```python
from build123d import *

# Parameters (mm, degrees)
F3_R           = 12.5
F3_R_2         = 9.5
F3_R_3         = 7.5
F4_DEPTH       = 5
F5_DEPTH       = 40
F6_START       = 8
F6_DEPTH       = 3
F7_START       = 14
F7_DEPTH       = 3
F8_R           = 1.49999
F9_R           = 1.49999
F10_R          = 4.99999
F14_R          = 2.5
F15_DEPTH      = 2.5
F15_DEPTH_BACK = 2.5
F16_SIZE       = 4.99999


# Not quite as in the source:
# - a fillet or chamfer is up to 0.001 mm smaller than in the source, because OpenCascade refuses the exact size


with BuildPart() as f4:
    # F3 (on Top) → F4 (new body)
    with BuildSketch(Plane.XY):
        Circle(F3_R)
        Circle(F3_R_2, mode=Mode.SUBTRACT)
        Circle(F3_R_2)
        Circle(F3_R_3, mode=Mode.SUBTRACT)
        Circle(F3_R_3)
    extrude(amount=F4_DEPTH)

    # F3 (on Top) → F5 (join)
    with BuildSketch(Plane.XY):
        Circle(F3_R_3)
    extrude(amount=F5_DEPTH)

    # F3 (on Top) → F6 (join)
    with BuildSketch(Plane.XY.offset(F6_START)):
        Circle(F3_R_2)
        Circle(F3_R_3, mode=Mode.SUBTRACT)
    extrude(amount=F6_DEPTH)

    # F3 (on Top) → F7 (join)
    with BuildSketch(Plane.XY.offset(F7_START)):
        Circle(F3_R_2)
        Circle(F3_R_3, mode=Mode.SUBTRACT)
    extrude(amount=F7_DEPTH)

    # F8 (radius 1.5 in the source; OpenCascade refuses exactly that, so slightly less here)
    f8_edges = [f4.edges().sort_by_distance(p)[0] for p in [
        (-9.5, 0, 8),
        (-9.5, 0, 11),
    ]]
    fillet(f8_edges, radius=F8_R)

    # F9 (radius 1.5 in the source; OpenCascade refuses exactly that, so slightly less here)
    f9_edges = [f4.edges().sort_by_distance(p)[0] for p in [
        (-9.5, 0, 14),
        (-9.5, 0, 17),
    ]]
    fillet(f9_edges, radius=F9_R)

    # F10 (radius 5 in the source; OpenCascade refuses exactly that, so slightly less here)
    f10_edges = [f4.edges().sort_by_distance(p)[0] for p in [
        (-12.5, 0, 5),
    ]]
    fillet(f10_edges, radius=F10_R)

    # F14 (on Front) → F15 (join, two sides)
    with BuildSketch(Plane.XZ) as f15_sk:
        Polygon((-2.5, 50), (-2.5, 40), (2.5, 40), (2.5, 50), (7.5, 50), (7.5, 55), (2.5, 55), (2.5, 60), (-2.5, 60), (-2.5, 55), (-7.5, 55), (-7.5, 50), align=None)
        with Locations((0, 50.75)):
            Circle(F14_R, mode=Mode.SUBTRACT)
    extrude(amount=F15_DEPTH)
    extrude(f15_sk.sketch, amount=-F15_DEPTH_BACK)

    # F16 (size 5 in the source; OpenCascade refuses exactly that, so slightly less here)
    f16_edges = [f4.edges().sort_by_distance(p)[0] for p in [
        (-2.5, 0, 50),
        (2.5, 0, 50),
    ]]
    chamfer(f16_edges, length=F16_SIZE)


solid = f4.part
```
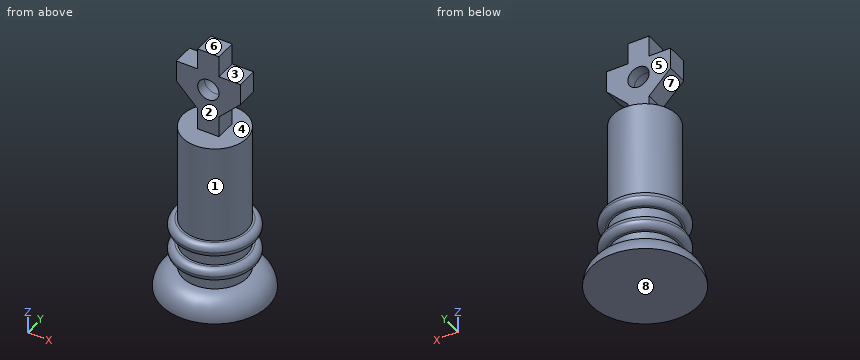
Design review of the part built by this model. Coordinates are the model's own, in mm. Face numbers are marked on the shaded views. A direction names the side the tool comes from. Coordinates: 2 decimals unless noted, no trailing zeros. Order: outer loops, then holes, each group sorted by start corner. A loop starts at its lowest first (then second) coordinate and runs counter-clockwise, first axis right, second up.
1) Wall thickness on line 1 along Z through (x, y) = (0, -1.85); line 2 along Z through (x, y) = (-1.5, -7.75); line 3 along X through (y, z) = (2.25, 45): over which ranges is each line inside the solid? List them lowest first.
2) Mouldability with a two-part tool opening along Z and no side actions: class the marked faces 1, 2 and 3 as +Z half, -Z half, draft (parallel to the pull), parting line (faces both ways), or undercut.
3) Take a section at B-B, the plane z = 43. Give the boundary of the cut face in (x, y), and give its area (3 significant figures).
4) Clearance check with flat-ended pins moving along their axes: pin 1 (5.5 mm diameter, centred on y = -0.5, z = 43.5, fed in from -X); pin 2 (7.5 mm diameter, centred on x = -0.5, z = 47.5, fed in from -Y); pin 3 (6 mm diameter, centred on y = -0.5, z = 17.5, fed in from +X); pin 4 (12 mm diameter, centred on x = 0, y = -6.5, fed in from +Z). State where each tip first meets the part, or that it passes through.
5) Take a section at A-A, the plane z = 50.75. Give the boundary of the cut face in (x, y).
6) For the marked faces 4, 5, 6, 7 and 8, list the 3-axis set-ups (+Z, -Z, +X, -X, +Y, -Y) from which the entire face can be reached by the end or side of a thin tool; tool diameter is ignored.
Returned:
1. line 1: z = 0 to 48.25, 53.25 to 60
1. line 2: z = 0 to 4.98, 8 to 11, 14 to 17
1. line 3: x = -2.5 to 2.5
2. face 1: undercut
2. face 2: draft
2. face 3: +Z half
3. outline: (-2.5, -2.5) - (2.5, -2.5) - (2.5, 2.5) - (-2.5, 2.5) - close
3. area: 25.0 mm2
4. pin 1: stops at x = -3.75
4. pin 2: stops at y = -2.5
4. pin 3: stops at x = 9.5
4. pin 4: stops at z = 60
5. outline: (-7.5, -2.5) - (-2.5, -2.5) - (-2.5, 2.5) - (-7.5, 2.5) - close; (2.5, -2.5) - (7.5, -2.5) - (7.5, 2.5) - (2.5, 2.5) - close
6. face 4: none
6. face 5: +Z, +X, -X, +Y
6. face 6: +Z, +X, -X, +Y, -Y
6. face 7: -X, +Y, -Y
6. face 8: -Z, +X, -X, +Y, -Y
